Could you check a few things on this model? Use its own coordinates, in mm. Face numbers are marked on the shaded views. Give positions to 0.01 mm unless a question says otherwise; leave off trailing zeros. Loops run counter-clockwise (first coordinate to the right, second up) from the corner with the lowest first, then second, coordinate; pieces in that order, holes last. Notation, with made-up numbers: (64.5, 61.25) - (81.5, 61.25) arc R14 ccw to (81.5, 83.25) - close; hole circle Ø9 at (15, 62). An arc over 180 degrees is marked (long way). Write each question's results on one line, items separated by ' | '. Start each with the question number.
(1) I need wall thicknesses on line 1 (X direction, y = -6, z = -1.5); line 2 (Z direction, x = 12, y = 0.5); line 3 (Y direction, x = 58.5, z = 2). Which ranges of each line are inside material? Lowest first, please.
(2) For pin 1 (3 mm diameter, centred on x = 56.5, y = -4.5, fed in from -Z); pin 2 (8 mm diameter, centred on x = 32, z = -2, fed in from +Y); pin 3 (1.5 mm diameter, centred on x = 42, z = -1, fed in from -Y); pin 4 (3.5 mm diameter, centred on x = 5, z = 0, fed in from -Y), each with a flat end and sliding along its axis, tell me the tip position at first contact or that it passes through.
(3) Suppose I cut it at C-C (x = 15). Please give me the cut outline in (y, z).
(4) If we mould it in two halves opening along Y, with no side actions, what happens to the marked faces 1, 2 and 3? For each: released by +Y, released by -Y, zero draft, split by the parting line, or undercut.
(5) Suppose I cut it at A-A (x = 58.5). Please give me the cut outline in (y, z).
(6) Suppose I cut it at B-B (x = 42.5). Please give me the cut outline in (y, z).
from build123d import *

# Parameters (mm, degrees)
F_12_0MM_DOWEL_HOLE1_D     = 12
F_12_0MM_DOWEL_HOLE1_DEPTH = 28
F_12_0MM_DOWEL_HOLE1_TIP   = 3.605163714
CUT_EXTRUDE2_DEPTH         = 3
M3X0_5_TAPPED_HOLE1_D      = 2.5
M3X0_5_TAPPED_HOLE1_DEPTH  = 6
M3X0_5_TAPPED_HOLE1_TIP    = 0.751075774
FILLET1_R                  = 0.5


with BuildPart() as part:
    # Sketch1 → Revolve1 (revolve)
    with BuildSketch(Plane.XY, mode=Mode.PRIVATE) as revolve1_sk:
        Polygon((0, 7.8), (0, 0), (64, 0), (64, 6), (50, 6), (50, 7.5), (32, 7.5), (32, 8.5), (16, 8.5), (9, 8.5), (9, 10), (1, 10), (1, 7.8), align=None)
    revolve(revolve1_sk.sketch.rotate(Axis((0, 0, 0), (1, 0, 0)), 90), axis=Axis((0, 0, 0), (1, 0, 0)))

    # Ø12.0mm Dowel Hole1
    with Locations(Plane.ZY):
        with Locations((0, 0)):
            Hole(F_12_0MM_DOWEL_HOLE1_D / 2, depth=F_12_0MM_DOWEL_HOLE1_DEPTH)
            with Locations((0, 0, -(F_12_0MM_DOWEL_HOLE1_DEPTH + F_12_0MM_DOWEL_HOLE1_TIP / 2))):  # 118° drill point
                Cone(0, F_12_0MM_DOWEL_HOLE1_D / 2, F_12_0MM_DOWEL_HOLE1_TIP, mode=Mode.SUBTRACT)

    # Sketch5 → Cut-Extrude2 (cut)
    with BuildSketch(Plane(origin=(0, -7.5, 0), x_dir=(-1, 0, 0), z_dir=(0, -1, 0))):
        with BuildLine():
            ThreePointArc((-46, -2.5), (-44.232233047, -1.767766953), (-43.5, 0))
            Line((-43.5, 0), (-48.5, 0))
            ThreePointArc((-48.5, -1.9e-08), (-47.767766946, -1.76776696), (-46, -2.5))
        make_face()
        with BuildLine():
            Line((-48.5, 0), (-43.5, 0))
            ThreePointArc((-43.5, 0), (-44.232233047, 1.767766953), (-46, 2.5))
            ThreePointArc((-46, 2.5), (-47.76776696, 1.767766946), (-48.5, -1.9e-08))
        make_face()
        with BuildLine():
            Line((-43.5, 0), (-38.5, 0))
            ThreePointArc((-38.5, 0), (-37.767766953, 1.767766953), (-36, 2.5))
            Line((-36, 2.5), (-46, 2.5))
            ThreePointArc((-46, 2.5), (-44.232233047, 1.767766953), (-43.5, 0))
        make_face()
        with BuildLine():
            ThreePointArc((-36, -2.5), (-37.767766953, -1.767766953), (-38.5, 0))
            Line((-38.5, 0), (-43.5, 0))
            ThreePointArc((-43.5, 0), (-44.232233047, -1.767766953), (-46, -2.5))
            Line((-46, -2.5), (-36, -2.5))
        make_face()
        with BuildLine():
            ThreePointArc((-36, -2.5), (-34.232233047, -1.767766953), (-33.5, 0))
            Line((-33.5, 0), (-38.5, 0))
            ThreePointArc((-38.5, 0), (-37.767766953, -1.767766953), (-36, -2.5))
        make_face()
        with BuildLine():
            Line((-38.5, 0), (-33.5, 0))
            ThreePointArc((-33.5, 0), (-34.232233047, 1.767766953), (-36, 2.5))
            ThreePointArc((-36, 2.5), (-37.767766953, 1.767766953), (-38.5, 0))
        make_face()
    extrude(amount=-CUT_EXTRUDE2_DEPTH, mode=Mode.SUBTRACT)

    # M3x0.5 Tapped Hole1
    with Locations(Plane(origin=(0, 8.5, 0), x_dir=(1, 0, 0), z_dir=(0, 1, 0))):
        with Locations((18, 0)):
            Hole(M3X0_5_TAPPED_HOLE1_D / 2, depth=M3X0_5_TAPPED_HOLE1_DEPTH)
            with Locations((0, 0, -(M3X0_5_TAPPED_HOLE1_DEPTH + M3X0_5_TAPPED_HOLE1_TIP / 2))):  # 118° drill point
                Cone(0, M3X0_5_TAPPED_HOLE1_D / 2, M3X0_5_TAPPED_HOLE1_TIP, mode=Mode.SUBTRACT)

    # Sketch11 → Ø4.0mm Dowel Hole1 (revolve, cut)
    with BuildSketch(Plane(origin=(5, 10, 0), x_dir=(0, 0, 1), z_dir=(1, 0, 0))):
        Polygon((0, 0), (0, 20), (2.025, 20), (2, 19.975), (2, 0.025), (2.025, 0), align=None)
    revolve(axis=Axis((5, 16.35, 0), (0, -1, 0)), mode=Mode.SUBTRACT)

    # Sketch12 → Ø4.0mm Dowel Hole2 (revolve, cut)
    with BuildSketch(Plane(origin=(58.5, 0, 6), x_dir=(0, -1, 0), z_dir=(1, 0, 0))):
        Polygon((0, 0), (0, 12), (2.025, 12), (2, 11.975), (2, 0.025), (2.025, 0), align=None)
    revolve(axis=Axis((58.5, 0, 12.35), (0, 0, -1)), mode=Mode.SUBTRACT)

    # Fillet1
    fillet1_edges = [part.edges().sort_by_distance(p)[0] for p in [
        (32, 0, -7.5),
        (50, 0, -6),
        (1, 0, -7.8),
        (9, 0, -8.5),
    ]]
    fillet(fillet1_edges, radius=FILLET1_R)


solid = part.part
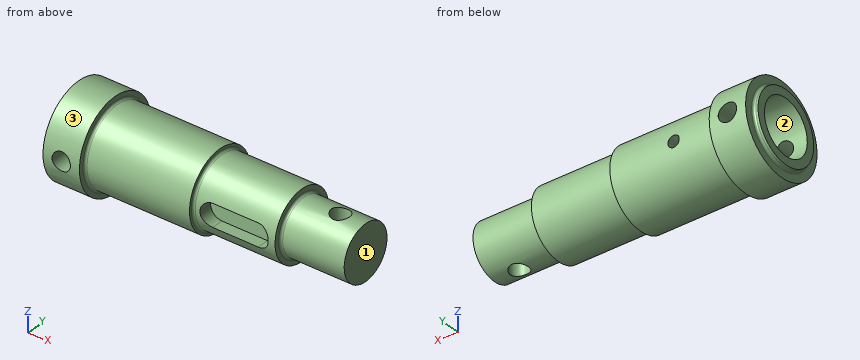
Output values:
1) line 1: 0 to 3.68, 6.32 to 34, 48 to 50.11 | line 2: -8.49 to -5.98, 5.98 to 8.49 | line 3: -5.66 to -2, 2 to 5.66
2) pin 1: z = -5.2 | pin 2: y = 8.5 | pin 3: y = -4.5 | pin 4: through
3) outline: circle Ø17 at (0, 0); hole circle Ø12 at (0, 0)
4) face 1: zero draft | face 2: undercut | face 3: split by the parting line
5) outline: (-2, -5.66) - (-2, 5.66) arc R6 ccw to start; (2, -5.66) arc R6 ccw to (2, 5.66) - close
6) outline: (-7.07, -2.5) arc R7.5 ccw (long way) to (-7.07, 2.5) - (-4.5, 2.5) - (-4.5, -2.5) - close
